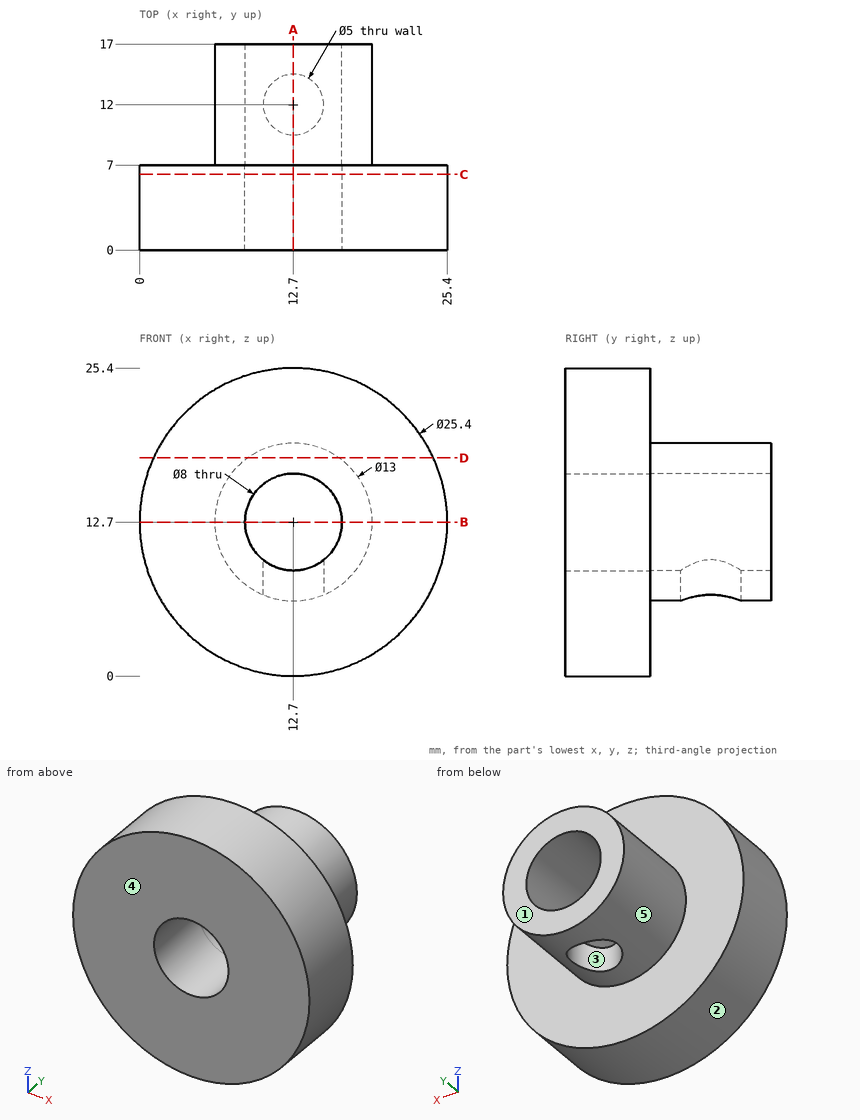
Check sheet for the drawn part. Datum: minimum x, y, z corner. Units: mm. A direction names the side the tool comes from. Coordinates: 2 decimals unless noted, no trailing zeros. Loops run counter-clockwise (first coordinate to the right, second up) from the corner with the lowest first, then second, coordinate; pieces in that order, holes last. Notation, with made-up numbers: (43.5, -16) -> (71.5, -16) arc R33 cw to (71.5, 17) -> close; hole circle Ø4 at (4.5, 2). An arc over 180 degrees is marked (long way). Answer in a Markdown table with one row per item.
1. Sectioned sample at C-C, the plane y = 6.25. Record the boundary of the cut face in (x, z).
Check values:
| item | result |
|---|---|
| outline | circle Ø25.4 at (12.7, 12.7); hole circle Ø8 at (12.7, 12.7) |
2. Go/stop test with flat-tipped pins: pin 1 (6 mm diameter, centred on x = 12.7, y = 12, fed in from -Z); pin 2 (4 mm diameter, centred on x = 5.5, y = 3, fed in from +Z); pin 3 (3 mm diameter, centred on y = 7.5, z = 8.5, fed in from +X); pin 4 (5 mm diameter, centred on x = 12.7, z = 12.7, fed in from -Y). Record where each tip stops, or that it passes through.
Check values:
| item | result |
|---|---|
| pin 1 | stops at z = 6.2 |
| pin 2 | stops at z = 24.29 |
| pin 3 | stops at x = 25.09 |
| pin 4 | passes through |
3. Release check for a two-part mould opening along Y. For the marked faces 1, 2 and 3 record: released by +Y, released by -Y, zero draft, split by the parting line, or undercut.
Check values:
| item | result |
|---|---|
| face 1 | released by +Y |
| face 2 | zero draft |
| face 3 | undercut |
4. Sectioned sample at A-A, the plane x = 12.7. Record the boundary of the cut face in (y, z), then the cut area to 3 significant figures.
Check values:
| item | result |
|---|---|
| outline | (0, 0) -> (7, 0) -> (7, 6.2) -> (9.5, 6.2) -> (9.5, 8.7) -> (0, 8.7) -> close; (0, 16.7) -> (17, 16.7) -> (17, 19.2) -> (7, 19.2) -> (7, 25.4) -> (0, 25.4) -> close; (14.5, 6.2) -> (17, 6.2) -> (17, 8.7) -> (14.5, 8.7) -> close |
| area | 159 mm2 |
5. Access from +Z, -Z, +X, -X, +Y, -Y to the whole of each face (thin tool, end or side, straight path). Record for the marked faces 4 and 5.
Check values:
| item | result |
|---|---|
| face 4 | +Z, -Z, +X, -X, -Y |
| face 5 | +Y |
6. Material ranges on line 1 along Z through (x, y) = (12.7, 3); line 2 along Y through (x, z) = (12.7, 8.05); line 3 along Y through (x, z) = (5.25, 16), recorded low to high. Write a range as [from, to].
Check values:
| item | result |
|---|---|
| line 1 | z = [0, 8.7], [16.7, 25.4] |
| line 2 | y = [0, 9.5], [14.5, 17] |
| line 3 | y = [0, 7] |
7. Sectioned sample at B-B, the plane z = 12.7. Record the boundary of the cut face in (x, y).
Check values:
| item | result |
|---|---|
| outline | (0, 0) -> (8.7, 0) -> (8.7, 17) -> (6.2, 17) -> (6.2, 7) -> (0, 7) -> close; (16.7, 0) -> (25.4, 0) -> (25.4, 7) -> (19.2, 7) -> (19.2, 17) -> (16.7, 17) -> close |
8. Sectioned sample at D-D, the plane z = 18. Record the boundary of the cut face in (x, y), then the cut area to 3 significant figures.
Check values:
| item | result |
|---|---|
| outline | (1.16, 0) -> (24.24, 0) -> (24.24, 7) -> (16.46, 7) -> (16.46, 17) -> (8.94, 17) -> (8.94, 7) -> (1.16, 7) -> close |
| area | 237 mm2 |
